Part model, mm, in its own coordinate system. Face numbers are marked on the shaded views. Give positions to 0.01 mm unless a question says otherwise; leave off trailing zeros. Loops run counter-clockwise (first coordinate to the right, second up) from the corner with the lowest first, then second, coordinate; pieces in that order, holes last. Notation, with made-up numbers: (69.5, 49) -> (123.5, 49) arc R29 ccw to (123.5, 83) -> close; hole circle Ø3 at (64, 50.25). An arc over 180 degrees is marked (long way). One line per question, with ' | ' between items.
```python
from build123d import *

# Parameters (mm, degrees)
F0_R     = 31.75
F0_R_2   = 25.4
F1_DEPTH = 6.35
F2_R     = 31.75
F3_DEPTH = 2.54


with BuildPart() as f1:
    # F0 (on Top) → F1 (new body)
    with BuildSketch(Plane.XY):
        Circle(F0_R)
        Circle(F0_R_2, mode=Mode.SUBTRACT)
    extrude(amount=F1_DEPTH)

    # F2 (on face) → F3 (join)
    with BuildSketch(Plane.XY.offset(6.35)):
        Circle(F2_R)
    extrude(amount=F3_DEPTH)

    # F4 (on Front) → F5 (revolve)
    with BuildSketch(Plane.XZ):
        with BuildLine():
            Line((-53.444212, 89.853903), (-31.75, 8.89))
            Line((-31.75, 8.89), (-29.120399, 8.89))
            Line((-29.120399, 8.89), (-51.472011, 92.307354))
            Line((-51.472011, 92.307354), (-51.561613, 92.307354))
            ThreePointArc((-51.561613, 92.307354), (-56.11673, 93.853608), (-53.444212, 89.853903))
        make_face()
    revolve(axis=Axis((0, 0, 53.792427), (0, 0, 1)))


solid = f1.part
```
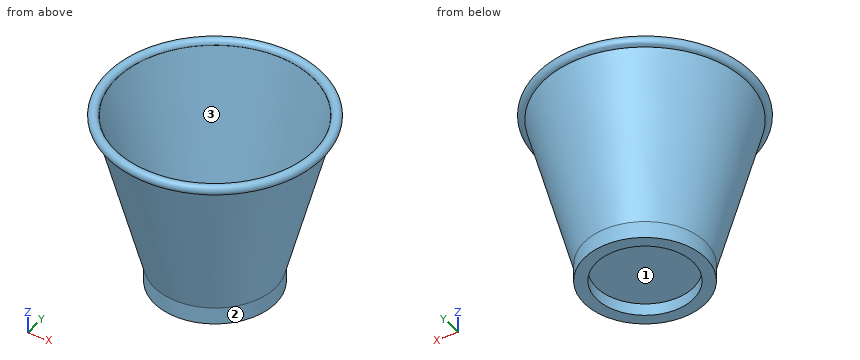
1) Saw through at D-D (z = 57). Give the cut face in (x, y), and give its area (3 significant figures).
Found:
outline: circle Ø89.28 at (0, 0); hole circle Ø84.02 at (0, 0) | area: 716 mm2
2) Pin check, flat tips, straight feed: P1, Ø3, axis at y = 11, z = 26.5, coming from the +X side; P2, Ø1, axis at x = 20, z = 47, coming from the -Y side; P3, Ø1.5, axis at y = -42, z = 59.5, coming from the +X side. Stop position of each tip, or through.
Found:
P1: x = 35.38 | P2: y = -37.2 | P3: x = 18.82
3) Drill centre lines: line 1 (Y direction, x = 0, z = 4); line 2 (Z direction, x = 9, y = -21.5); line 3 (X direction, y = -18.5, z = 27). Where is each one in solid material? Low to high.
Found:
line 1: -31.75 to -25.4, 25.4 to 31.75 | line 2: 6.35 to 8.89 | line 3: -31.58 to -28.49, 28.49 to 31.58
4) Saw through at A-A (y = 0). Give the cut face in (x, z), and give its area (3 significant figures).
Found:
outline: (-53.44, 89.85) -> (-31.75, 8.89) -> (-31.75, 0) -> (-25.4, 0) -> (-25.4, 6.35) -> (25.4, 6.35) -> (25.4, 0) -> (31.75, 0) -> (31.75, 8.89) -> (53.44, 89.85) arc R2.54 ccw (long way) to (51.56, 92.31) -> (51.47, 92.31) -> (29.12, 8.89) -> (-29.12, 8.89) -> (-51.47, 92.31) -> (-51.56, 92.31) arc R2.54 ccw (long way) to start | area: 713 mm2
5) Saw through at C-C (z = 11). Give the cut face in (x, y).
Found:
outline: circle Ø64.63 at (0, 0); hole circle Ø59.37 at (0, 0)
6) Pull direction Y, two halves, no side cores. Call the marked faces 1, 2 and 3: pulls with the +Y half, pulls with the -Y half, needs draft (parallel to the pull), parting line crosses it, or undercut.
Found:
face 1: undercut | face 2: parting line crosses it | face 3: undercut
